The drawing under review shows one solid part. Ordinate dimensions are in mm from its lowest x, y, z. A direction names the side the tool comes from. Coordinates: 2 decimals unless noted, no trailing zeros. Order: outer loops, then holes, each group sorted by start corner. A loop starts at its lowest first (then second) coordinate and runs counter-clockwise, first axis right, second up.
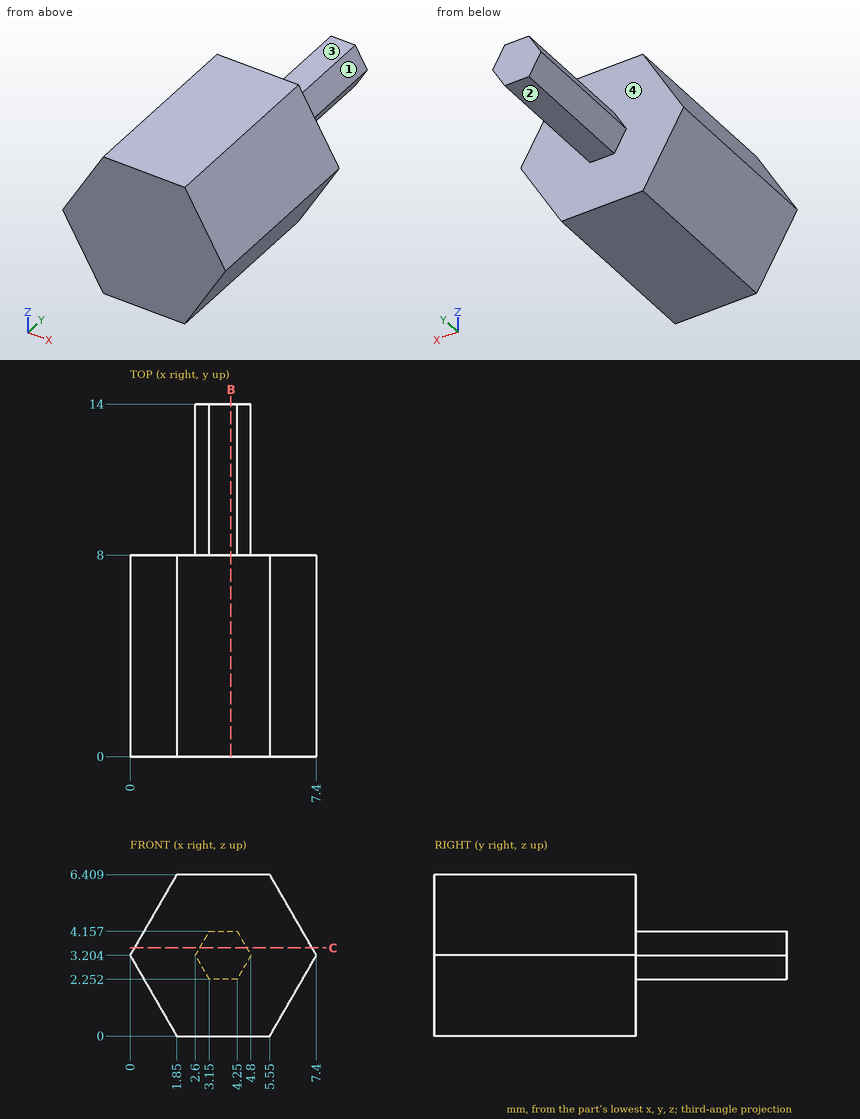
1. Insertion check: pin 1 (1.2 mm diameter, centred on x = 3.5, y = 11.5, fed in from +Z); pin 2 (1.2 mm diameter, centred on x = 3.5, y = 12, fed in from -Z); pin 3 (3 mm diameter, centred on y = 3.5, z = 4, fed in from +X); pin 4 (3 mm diameter, centred on x = 1, y = 6, fed in from +Z). Each pin has a flat end and moves straight along its axis. Give the tip position at first contact, or say it passes through.
2. For the marked faces 1, 2, 3 and 4, list the 3-axis set-ups (+Z, -Z, +X, -X, +Y, -Y) from which the entire face can be reached by the end or side of a thin tool; tool diameter is ignored.
3. Add section C-C (z = 3.5). Give the boundary of the cut face in (x, y).
4. To check wall thickness, follow line 1 (Y direction, x = 4.5, z = 5); line 2 (Z direction, x = 2.75, y = 10.75) (1 decimal); line 3 (X direction, y = 2.25, z = 2.5) (1 decimal). State the ranges of each line that lie inside material, in increasing order.
5. Add section B-B (x = 4). Give the boundary of the cut face in (y, z).
Solution:
1. pin 1: stops at z = 4.16
1. pin 2: stops at z = 2.25
1. pin 3: stops at x = 7.4
1. pin 4: stops at z = 6.41
2. face 1: +Z, +X, +Y
2. face 2: -Z, +X, -X, +Y
2. face 3: +Z, +X, -X, +Y
2. face 4: +Y
3. outline: (0.17, 0) - (7.23, 0) - (7.23, 8) - (4.63, 8) - (4.63, 14) - (2.77, 14) - (2.77, 8) - (0.17, 8) - close
4. line 1: y = 0 to 8
4. line 2: z = 2.9 to 3.5
4. line 3: x = 0.4 to 7
5. outline: (0, 0) - (8, 0) - (8, 2.25) - (14, 2.25) - (14, 4.16) - (8, 4.16) - (8, 6.41) - (0, 6.41) - close
